from build123d import *

# Parameters (mm, degrees)
SKETCH1_R           = 51.054
SKETCH1_R_2         = 49.657
BOSS_EXTRUDE1_DEPTH = 609.6
SKETCH2_R           = 1.984375
CUT_EXTRUDE1_DEPTH  = 12.7
CIRPATTERN1_COUNT   = 4


with BuildPart() as part:
    # Sketch1 → Boss-Extrude1 (new body)
    with BuildSketch(Plane(origin=(0, 0, 0), x_dir=(1, 0, 0), z_dir=(0, 1, 0))):
        with Locations(Location((0, 0, 0), (0, 0, 90))):
            Circle(SKETCH1_R)
        with Locations(Location((0, 0, 0), (0, 0, 90))):
            Circle(SKETCH1_R_2, mode=Mode.SUBTRACT)
    extrude(amount=BOSS_EXTRUDE1_DEPTH)

    # Sketch2 → Cut-Extrude1 (cut)
    with BuildSketch(Plane(origin=(122.899951256, 815.595371644, -42.551362721), x_dir=(-0.9976910351931784, 0, -0.067916112191174), z_dir=(0.067916112191174, 0, -0.9976910351931785))):
        with Locations((119.72625647, -256.795371644)):
            Circle(SKETCH2_R)
    cut_extrude1 = extrude(amount=-CUT_EXTRUDE1_DEPTH, mode=Mode.SUBTRACT)

    # CirPattern1: Cut-Extrude1 ×4 about axis
    cirpattern1_axis = Axis((0, 0, 0), (0, 1, 0))
    for i in range(1, CIRPATTERN1_COUNT):
        add(cut_extrude1.rotate(cirpattern1_axis, i * 360 / CIRPATTERN1_COUNT), mode=Mode.SUBTRACT)


solid = part.part
Work out the finished part from the listing and answer in its coordinate system (mm). Coordinates: 2 decimals unless noted, no trailing zeros. Order: outer loops, then holes, each group sorted by start corner. A loop starts at its lowest first (then second) coordinate and runs counter-clockwise, first axis right, second up. Notation, with made-up numbers: (30.5, -10.75) - (88.5, -10.75) arc R12 ccw to (88.5, 0.25) - close; hole circle Ø7 at (73, -28.75). An arc over 180 degrees is marked (long way). Put each result on its own line as item: value. Start each with the question number.
1) Find the intervals of material crossed by line 1 (X direction, y = 409.5, z = 0); line 2 (Z direction, x = -5.5, y = 66.5); line 3 (X direction, y = 214.5, z = 22), in increasing order. Write a range as from..to.
2) For a pull along Z with two mould halves and no side action, classify faces 1 (the cylindrical face through (19.554, 300.533, -47.161)), 2 (the flat face through (49, 609.6, -11)), 3 (the cylindrical face through (-49.234, 300.533, 6.464)) as released by +Z, released by -Z, zero draft, split by the parting line, or undercut.
3) Find section C-C (y = 373). Give the vertices of the cut face in (x, z), plus the area to 3 significant figures.
4) Find section B-B (z = 33.5). Give the vertices of the cut face in (x, y).
5) Find section A-A (x = 42). Give the vertices of the cut face in (y, z).
6) Flat-ended cylindrical pins translate along their axes: pin 1 (1.5 mm diameter, centred on x = -28, y = 81, fed in from +Z); pin 2 (8 mm diameter, centred on y = 517, z = -4, fed in from +X); pin 3 (2 mm diameter, centred on y = 521, z = -34.5, fed in from +X). Find the tip coordinate at first contact, or state that the pin passes through.
Results list:
1. line 1: x = -51.05..-49.66, 49.66..51.05
1. line 2: z = -50.76..-49.35, 49.35..50.76
1. line 3: x = -46.07..-44.52, 44.52..46.07
2. face 1: split by the parting line
2. face 2: zero draft
2. face 3: undercut
3. outline: circle Ø102.11 at (0, 0); hole circle Ø99.31 at (0, 0)
3. area: 442 mm^2
4. outline: (-38.53, 0) - (-36.65, 0) - (-36.65, 609.6) - (-38.53, 609.6) - close; (36.65, 0) - (38.53, 0) - (38.53, 609.6) - (36.65, 609.6) - close
5. outline: (0, -29.03) - (609.6, -29.03) - (609.6, -26.49) - (0, -26.49) - close; (0, 26.49) - (609.6, 26.49) - (609.6, 29.03) - (0, 29.03) - close
6. pin 1: stops at z = 43.17
6. pin 2: stops at x = 51.05
6. pin 3: stops at x = 38.53
